Read the model definition and answer for the solid it produces. Units are mm, in the model's axes. A direction names the side the tool comes from. Give positions to 0.01 mm unless a question says otherwise; leave off trailing zeros. Order: outer loops, then holes, each group sorted by start corner. A loop starts at its lowest first (then second) coordinate and runs counter-clockwise, first axis right, second up.
Item 1: The mould has two halves that part along Z. Classify faces 5 (the face through (25.578, 0.279, 63.497)), 6 (the face through (101.594, -0.559, 12.522)), 7 (the face through (25.6, -0.8, 57.1)): +Z half, -Z half, draft (parallel to the pull), parting line (faces both ways), or undercut.
Item 2: A cutting plane is placed at D-D (x = -73). Write down the section's boundary in (y, z).
Item 3: A cutting plane is placed at C-C (z = 8). Write down the section's boundary in (x, y), plus the area to 3 significant figures.
Item 4: Find the intervals of material crossed by line 1 along X through (y, z) = (-11, 54.5); line 2 along Y through (x, z) = (-76.2, 16.25); line 3 along Y through (x, z) = (-26.25, 50.8), in increasing order.
Item 5: A cutting plane is placed at A-A (y = -4). Write down the section's boundary in (x, z).
Item 6: Which of the six approach directions +Z, -Z, +X, -X, +Y, -Y give full straight-line access (tool end or side, diameter ignored) to faces 1 (the face through (1, -12.7, 30)), 2 (the face through (1, 12.7, 29)), 3 (the face through (-12.7, 0, 58)), 4 (the face through (-38.1, 0, 40))?
Item 7: A cutting plane is placed at B-B (x = 23.5). Write down the section's boundary in (y, z).
Item 8: Given pin 1 Ø20.5 at (y, z) = (0, 50.8) entering from +X; pin 2 Ø10 at (y, z) = (0.5, 47.5) entering from -X; pin 3 Ø10 at (x, y) = (-65, -6) entering from -Z; pin 4 Ø5 at (x, y) = (61.5, 9.5) entering from +Z, each flat-ended and moving along its own axis, determine where each tip first touches the part or whether it passes through.
from build123d import *

# Parameters (mm, degrees)
F0_R          = 12.7
F1_DEPTH      = 25.4
F2_R          = 6.35
F3_DEPTH      = 38.1
F3_DEPTH_BACK = 38.1
F5_DEPTH      = 25.4
F5_DEPTH_BACK = 25.4


with BuildPart() as f1:
    # F0 (on Top) → F1 (new body)
    with BuildSketch(Plane.XY):
        with BuildLine():
            Line((76.2, 25.4), (-76.2, 25.4))
            ThreePointArc((-76.2, 25.4), (-101.6, 0), (-76.2, -25.4))
            Line((-76.2, -25.4), (76.2, -25.4))
            ThreePointArc((76.2, -25.4), (101.6, 0), (76.2, 25.4))
        make_face()
        with Locations((-76.2, 0)):
            Circle(F0_R, mode=Mode.SUBTRACT)
        with Locations((76.2, 0)):
            Circle(F0_R, mode=Mode.SUBTRACT)
    extrude(amount=F1_DEPTH)

    # F2 (on Right) → F3 (join, two sides)
    with BuildSketch(Plane.YZ) as f3_sk:
        with BuildLine():
            Line((-12.7, 50.8), (-12.7, 25.4))
            Line((-12.7, 25.4), (12.7, 25.4))
            Line((12.7, 25.4), (12.7, 50.8))
            ThreePointArc((12.7, 50.8), (0, 63.5), (-12.7, 50.8))
        make_face()
        with Locations((0, 50.8)):
            Circle(F2_R, mode=Mode.SUBTRACT)
    extrude(amount=F3_DEPTH)
    extrude(f3_sk.sketch, amount=-F3_DEPTH_BACK)

    # F4 (on Front) → F5 (cut, two sides)
    with BuildSketch(Plane.XZ) as f5_sk:
        with BuildLine():
            Line((12.7, 43.18), (12.7, 63.5))
            Line((12.7, 63.5), (-12.7, 63.5))
            Line((-12.7, 63.5), (-12.7, 43.18))
            ThreePointArc((-12.7, 43.18), (0, 30.48), (12.7, 43.18))
        make_face()
    extrude(amount=-F5_DEPTH, mode=Mode.SUBTRACT)
    extrude(f5_sk.sketch, amount=F5_DEPTH_BACK, mode=Mode.SUBTRACT)


solid = f1.part
Response values:
1. face 5: +Z half
1. face 6: draft
1. face 7: undercut
2. outline: (-25.4, 0) - (-12.29, 0) - (-12.29, 25.4) - (-25.4, 25.4) - close; (12.29, 0) - (25.4, 0) - (25.4, 25.4) - (12.29, 25.4) - close
3. outline: (-76.2, -25.4) - (76.2, -25.4) arc R25.4 ccw to (76.2, 25.4) - (-76.2, 25.4) arc R25.4 ccw to start; hole circle Ø25.4 at (-76.2, 0); hole circle Ø25.4 at (76.2, 0)
3. area: 8,760 mm2
4. line 1: x = -38.1 to -12.7, 12.7 to 38.1
4. line 2: y = -25.4 to -12.7, 12.7 to 25.4
4. line 3: y = -12.7 to -6.35, 6.35 to 12.7
5. outline: (-101.28, 0) - (-88.25, 0) - (-88.25, 25.4) - (-101.28, 25.4) - close; (-64.15, 0) - (64.15, 0) - (64.15, 25.4) - (38.1, 25.4) - (38.1, 45.87) - (12.7, 45.87) - (12.7, 43.18) arc R12.7 cw to (-12.7, 43.18) - (-12.7, 45.87) - (-38.1, 45.87) - (-38.1, 25.4) - (-64.15, 25.4) - close; (-38.1, 55.73) - (-12.7, 55.73) - (-12.7, 62.85) - (-38.1, 62.85) - close; (12.7, 55.73) - (38.1, 55.73) - (38.1, 62.85) - (12.7, 62.85) - close; (88.25, 0) - (101.28, 0) - (101.28, 25.4) - (88.25, 25.4) - close
6. face 1: +Z, +X, -X, -Y
6. face 2: +Z, +X, -X, +Y
6. face 3: +Z, +Y, -Y
6. face 4: +Z, -X, +Y, -Y
7. outline: (-25.4, 0) - (25.4, 0) - (25.4, 25.4) - (12.7, 25.4) - (12.7, 50.8) arc R12.7 ccw to (-12.7, 50.8) - (-12.7, 25.4) - (-25.4, 25.4) - close; hole circle Ø12.7 at (0, 50.8)
8. pin 1: stops at x = 38.1
8. pin 2: stops at x = -38.1
8. pin 3: stops at z = 0
8. pin 4: stops at z = 25.4
